from build123d import *

# Parameters (mm, degrees)
SKETCH_1_W                 = 22.72
SKETCH_1_H                 = 10
EXTRUDE_269_DEPTH          = 2
SKETCH_3_W                 = 2.4
SKETCH_3_H                 = 10
EXTRUDE_2_DEPTH            = 1.27
PATTERN_LINEAR_1_COUNT     = 3
PATTERN_LINEAR_1_PITCH     = 5.08
PATTERN_LINEAR_1_COL_COUNT = 3
PATTERN_LINEAR_1_COL_PITCH = 5.08
EXTRUDE_START              = 5
SKETCH_4_W                 = 22.72
SKETCH_4_H                 = 2
EXTRUDE_3_DEPTH            = 6.2
EXTRUDE_START_2            = -5
SKETCH_4_2_W               = 22.72
SKETCH_4_2_H               = 2
EXTRUDE_4_DEPTH            = 6.2
EXTRUDE_1_DEPTH            = 3.8
HOLE_WIZARD_M3_1_D         = 3.2


with BuildPart() as part:
    # 草图1 → Extrude 269 (new body)
    with BuildSketch(Plane(origin=(0, 0, 0), x_dir=(1, 0, 0), z_dir=(0, 1, 0))):
        Rectangle(SKETCH_1_W, SKETCH_1_H)
    extrude(amount=EXTRUDE_269_DEPTH)

    # 草图3 → 凸台-拉伸2 (add)
    with BuildSketch(Plane(origin=(0, 2, 0), x_dir=(1, 0, 0), z_dir=(0, 1, 0))):
        Rectangle(SKETCH_3_W, SKETCH_3_H)
    extrude_2 = extrude(amount=EXTRUDE_2_DEPTH)

    # 阵列(线性)1: 凸台-拉伸2 ×3
    with Locations(*[(i * PATTERN_LINEAR_1_PITCH, 0, 0) for i in range(1, PATTERN_LINEAR_1_COUNT)]):
        add(extrude_2)

    # 阵列(线性)1 col: 凸台-拉伸2 ×3
    with Locations(*[(-i * PATTERN_LINEAR_1_COL_PITCH, 0, 0) for i in range(1, PATTERN_LINEAR_1_COL_COUNT)]):
        add(extrude_2)

    # 草图4 → 凸台-拉伸3 (add)
    with BuildSketch(Plane.XY.offset(EXTRUDE_START)):
        with Locations((0, 1)):
            Rectangle(SKETCH_4_W, SKETCH_4_H)
    extrude(amount=EXTRUDE_3_DEPTH)

    # 草图4<2> → 凸台-拉伸4 (add)
    with BuildSketch(Plane.XY.offset(EXTRUDE_START_2)):
        with Locations((0, 1)):
            Rectangle(SKETCH_4_2_W, SKETCH_4_2_H)
    extrude(amount=-EXTRUDE_4_DEPTH)

    # 草图5 → 拉伸-薄壁1 (add)
    with BuildSketch(Plane.XZ):
        Polygon((7.007942216, 11.27238461), (3.303977501, 9.143070466), (3.296035285, 4.870685856), (6.992057784, 2.72761539), (10.696022499, 4.856929534), (10.703964715, 9.129314144), align=None)
        Polygon((7.00622498, 10.348625775), (4.103117501, 8.679703878), (4.096892521, 5.331078103), (6.99377502, 3.651374225), (9.896882499, 5.320296122), (9.903107479, 8.668921897), align=None, mode=Mode.SUBTRACT)
    extrude_1 = extrude(amount=EXTRUDE_1_DEPTH)

    # 草图阵列1: 拉伸-薄壁1 at 3 more places
    with Locations((0, 0, -14), (-14, 0, -14), (-14, 0, 0)):
        add(extrude_1)

    # M3 间隙孔1 (through all)
    with Locations(Plane(origin=(0, 2, 0), x_dir=(1, 0, 0), z_dir=(0, 1, 0))):
        with Locations((7, -7)):
            hole_wizard_m3_1 = Hole(HOLE_WIZARD_M3_1_D / 2)

    # 草图阵列2: M3 间隙孔1 at 3 more places
    with Locations((0, 0, -14), (-14, 0, -14), (-14, 0, 0)):
        add(hole_wizard_m3_1, mode=Mode.SUBTRACT)


solid = part.part
Could you check a few things on this model? Use its own coordinates, in mm. A direction names the side the tool comes from. Round coordinates to 2 decimals unless told otherwise and drop trailing zeros. Order: outer loops, then holes, each group sorted by start corner. A loop starts at its lowest first (then second) coordinate and runs counter-clockwise, first axis right, second up.
(1) Imagine slicing it at B-B (z = -7.5). Write out the boundary of the cut face in (x, y), plus the area to 3 significant figures.
Response values:
outline: (-11.36, 0) - (-10.7, 0) - (-10.7, -3.8) - (-9.9, -3.8) - (-9.9, 0) - (-8.52, 0) - (-8.52, 2) - (-11.36, 2) - close; (-5.48, 0) - (-4.1, 0) - (-4.1, -3.8) - (-3.3, -3.8) - (-3.3, 0) - (3.3, 0) - (3.3, -3.8) - (4.1, -3.8) - (4.1, 0) - (5.48, 0) - (5.48, 2) - (-5.48, 2) - close; (8.52, 0) - (9.9, 0) - (9.9, -3.8) - (10.7, -3.8) - (10.7, 0) - (11.36, 0) - (11.36, 2) - (8.52, 2) - close
area: 45.4 mm2
(2) If we mould it in two halves opening along Z, with no side actions, what happens to faces 1 (the flat face through (-6, -3.8, 4)), 2 (the flat face through (-5.53, -1.87, -4.5)), 3 (the flat face through (8.882, -1.873, 10.186))? For each: released by +Z, released by -Z, zero draft, split by the parting line, or undercut.
Response values:
face 1: zero draft
face 2: undercut
face 3: released by +Z
(3) Please list where these lines run through material, in increasing order: line 1 along X through (y, z) = (1, 7); line 2 along X through (y, z) = (2.5, -3.25); line 3 along Z through (x, y) = (7, 0.5).
Response values:
line 1: x = -11.36 to -8.6, -5.4 to 5.4, 8.6 to 11.36
line 2: x = -11.36 to -8.96, -6.28 to -3.88, -1.2 to 1.2, 3.88 to 6.28, 8.96 to 11.36
line 3: z = -11.2 to -8.6, -5.4 to 5.4, 8.6 to 11.2
(4) Imagine slicing it at A-A (y = 0.5). Write out the boundary of the cut face in (x, z), plus the area to 3 significant figures.
Response values:
outline: (-11.36, -11.2) - (11.36, -11.2) - (11.36, 11.2) - (-11.36, 11.2) - close; hole circle Ø3.2 at (-7, -7); hole circle Ø3.2 at (-7, 7); hole circle Ø3.2 at (7, -7); hole circle Ø3.2 at (7, 7)
area: 477 mm2
(5) Imagine slicing it at C-C (y = 2.5). Write out the boundary of the cut face in (x, z), plus the area to 3 significant figures.
Response values:
outline: (-11.36, -5) - (-8.96, -5) - (-8.96, 5) - (-11.36, 5) - close; (-6.28, -5) - (-3.88, -5) - (-3.88, 5) - (-6.28, 5) - close; (-1.2, -5) - (1.2, -5) - (1.2, 5) - (-1.2, 5) - close; (3.88, -5) - (6.28, -5) - (6.28, 5) - (3.88, 5) - close; (8.96, -5) - (11.36, -5) - (11.36, 5) - (8.96, 5) - close
area: 120 mm2
(6) Which directions (+Z, -Z, +X, -X, +Y, -Y) give clear straight access to the entire face, cutting with the end or side of a thin tool? Please do faces 4 (the flat face through (5.18, -1.87, -3.78)), 5 (the flat face through (5, 3, -5)), 6 (the flat face through (5, 3, 5)).
Response values:
face 4: -Y
face 5: -Z, +X, -X, +Y
face 6: +Z, +X, -X, +Y
(7) I'm going to push flat-ended pins straight in: pin 1 (1.5 mm diameter, centred on x = 1, z = 6, fed in from -Y); pin 2 (2 mm diameter, centred on x = 4, y = 1, fed in from -Z); pin 3 (2 mm diameter, centred on x = -1, y = 1, fed in from +Z). Where does each tip first touch, or does it pass through?
Response values:
pin 1: stops at y = 0
pin 2: stops at z = -11.2
pin 3: stops at z = 11.2
(8) Imagine slicing it at D-D (x = 0.25). Write out the boundary of the cut face in (y, z).
Response values:
outline: (0, -11.2) - (2, -11.2) - (2, -5) - (3.27, -5) - (3.27, 5) - (2, 5) - (2, 11.2) - (0, 11.2) - close
